The listing builds one solid part. Answer for the finished solid, in the listing's coordinates (mm). Face numbers are marked on the shaded views. A direction names the side the tool comes from. Coordinates: 2 decimals unless noted, no trailing zeros. Order: outer loops, then holes, each group sorted by start corner. A loop starts at its lowest first (then second) coordinate and runs counter-clockwise, first axis right, second up. Notation, with made-up numbers: (42.25, 6.5) -> (76.25, 6.5) arc R19 ccw to (76.25, 10.5) -> close; hole circle Ø9 at (-14, -32). An arc over 180 degrees is marked (long way). Answer in a Markdown table with one row per item.
Autodesk Inventor part; units mm, degrees
ref_plane "YZ Plane" through (0, 0, 0) normal (1, 0, 0) x (0, 1, 0)
ref_plane "XZ Plane" through (0, 0, 0) normal (0, 1, 0) x (-1, 0, 0)
ref_plane "XY Plane" through (0, 0, 0) normal (0, 0, 1) x (1, 0, 0)
sketch "Sketch1" plane through (0, 0, 0) normal (0, 1, 0) x (-1, 0, 0)
  line L0 (-9.6397, 29.7296) -> (10.3603, 29.7296)
  line L1 (12.3603, 29.7296) -> (12.3603, 36.7296)
  line L2 (12.3603, 36.7296) -> (-9.6397, 36.7296)
  line L3 (-9.6397, 36.7296) -> (-9.6397, 29.7296)
  line L4 (12.3603, 36.7296) -> (8.0662, 36.7296)
  line L5 (8.0662, -18.2704) -> (12.3603, -18.2704)
  line L6 (12.3603, -18.2704) -> (-9.6397, -18.2704)
  line L7 (-9.6397, -18.2704) -> (-9.6397, -11.2704)
  line L8 (-9.6397, -11.2704) -> (10.3603, -11.2704)
  line L9 (12.3603, -11.2704) -> (12.3603, -18.2704)
  line L10 (12.3603, -7.7704) -> (22.3603, -7.7704)
  line L11 (22.3603, -7.7704) -> (22.3603, 16.2296)
  line L12 (22.3603, 16.2296) -> (12.3603, 16.2296)
  line L13 (12.3603, -18.2704) -> (12.3603, -7.7704)
  line L14 (12.3603, 16.2296) -> (12.3603, 36.7296)
  line L15 (10.3603, 14.2296) -> (20.3603, 14.2296)
  line L16 (20.3603, 14.2296) -> (20.3603, -5.7704)
  line L17 (20.3603, -5.7704) -> (10.3603, -5.7704)
  line L18 (10.3603, 22.4354) -> (10.3603, 14.2296)
  line L19 (10.3603, -5.7704) -> (10.3603, -4.741)
  line L20 (10.3603, 29.7296) -> (10.3603, 14.2296)
  line L21 (10.3603, -5.7704) -> (10.3603, -11.2704)
  point P0 (0, 0)
  dimension "wall" = 2
  dimension "d1" = 2
  dimension "d2" = 2
  dimension "d3" = 2
  dimension "d4" = 2
  dimension "d5" = 7
  dimension "d6" = 7
  dimension "d7" = 20
  dimension "d8" = 20
  dimension "d9" = 41
  dimension "d10" = 5.5
  dimension "d11" = 20
  dimension "d12" = 10
extrude "Extrusion1" add sketch "Sketch1" along normal blind 10
sketch "Sketch2" plane through (0, 10, 0) normal (0, 1, 0) x (1, 0, 0)
  line L0 (-10.3603, -29.7296) -> (-10.3603, -14.2296) construction
  line L1 (-12.3603, -36.7296) -> (9.6397, -36.7296) construction
  line L2 (9.6397, 18.2704) -> (-12.3603, 18.2704) construction
  line L3 (3.8669, 14.7392) -> (-5.6603, 14.7392) construction
  line L4 (-5.6603, 14.7392) -> (-5.6603, -33.2296) construction
  line L5 (-5.6603, -33.2296) -> (3.8669, -33.2296) construction
  line L6 (3.8669, -33.2296) -> (3.8669, 14.7392) construction
  point P0 (0, 0)
  point P1 (3.8397, -33.2296)
  point P2 (-5.6603, 14.7704)
  dimension "d15" = 4.7
  dimension "d16" = 9.5
  dimension "d17" = 48
  dimension "d18" = 3.5
  dimension "d19" = 3.5
hole "Hole1" at (-5.6603, 10, 33.2296) at (3.8397, 10, 33.2296) at (3.8669, 10, -14.7392) at (-5.6603, 10, -14.7704) direction (0, -1, 0) diameter 1.5 end through all
fillet "Fillet1" radius 2 8 edges at (9.6397, 5, 36.7296) (-12.3603, 5, 36.7296) (9.6397, 5, -18.2704) (-12.3603, 5, -18.2704) (-22.3603, 5, -7.7704) (-12.3603, 5, -7.7704) (-22.3603, 5, 16.2296) (-12.3603, 5, 16.2296)
equation "\"d1\" = wall"
equation "\"d2\" = wall"
equation "\"d3\" = wall"
equation "\"d4\" = wall"
equation "\"d6\" = d5"
equation "\"d8\" = d7"
properties part number "servo_bracket"
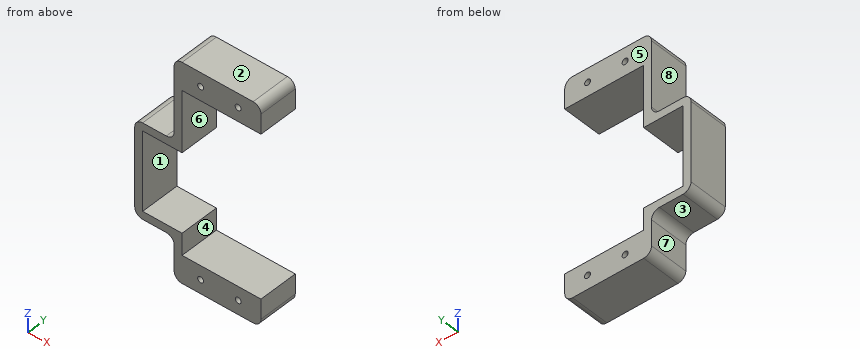
(1) A cutting plane is placed at A-A, the plane x = -19. Determine the outline of the cut face in (y, z).
Check values:
| item | result |
|---|---|
| outline | (0, -7.77) -> (10, -7.77) -> (10, -5.77) -> (0, -5.77) -> close; (0, 14.23) -> (10, 14.23) -> (10, 16.23) -> (0, 16.23) -> close |
(2) Flat-ended cylindrical pins translate along their axes: pin 1 (3 mm diameter, centred on y = 4, z = 7.5, fed in from +X); pin 2 (3 mm diameter, centred on x = -17, y = 5.5, fed in from -Z); pin 3 (1.2 mm diameter, centred on x = -5.66, z = -14.77, fed in from +Y); pin 4 (3 mm diameter, centred on x = -18, y = 3, fed in from +Z). Find the tip coordinate at first contact, or state that the pin passes through.
Check values:
| item | result |
|---|---|
| pin 1 | x = -20.36 |
| pin 2 | z = -7.77 |
| pin 3 | through |
| pin 4 | z = 16.23 |
(3) Find the intervals of material crossed by line 1 along Z through (x, y) = (5, 5.75); line 2 along Z through (x, y) = (-18.5, 2.5); line 3 along X through (y, z) = (3, 33), in increasing order. Write a range as from..to.
Check values:
| item | result |
|---|---|
| line 1 | -18.27..-11.27, 29.73..36.73 |
| line 2 | -7.77..-5.77, 14.23..16.23 |
| line 3 | -12.36..-6.37, -4.95..3.13, 4.55..9.64 |
(4) For a pull along Z with two mould halves and no side action, classify the marked faces 1, 2, 3 and 4 as released by +Z, released by -Z, zero draft, split by the parting line, or undercut.
Check values:
| item | result |
|---|---|
| face 1 | undercut |
| face 2 | released by +Z |
| face 3 | released by -Z |
| face 4 | undercut |
(5) A cutting plane is placed at D-D, the plane z = -12. Determine the outline of the cut face in (x, y), then the cut area to 3 significant figures.
Check values:
| item | result |
|---|---|
| outline | (-12.36, 0) -> (9.64, 0) -> (9.64, 10) -> (-12.36, 10) -> close |
| area | 220 mm² |
(6) A cutting plane is placed at B-B, the plane y = 9. Determine the outline of the cut face in (x, z), then the cut area to 3 significant figures.
Check values:
| item | result |
|---|---|
| outline | (-22.36, -5.77) arc R2 ccw to (-20.36, -7.77) -> (-14.36, -7.77) arc R2 cw to (-12.36, -9.77) -> (-12.36, -16.27) arc R2 ccw to (-10.36, -18.27) -> (7.64, -18.27) arc R2 ccw to (9.64, -16.27) -> (9.64, -11.27) -> (-10.36, -11.27) -> (-10.36, -5.77) -> (-20.36, -5.77) -> (-20.36, 14.23) -> (-10.36, 14.23) -> (-10.36, 29.73) -> (9.64, 29.73) -> (9.64, 34.73) arc R2 ccw to (7.64, 36.73) -> (-10.36, 36.73) arc R2 ccw to (-12.36, 34.73) -> (-12.36, 18.23) arc R2 cw to (-14.36, 16.23) -> (-20.36, 16.23) arc R2 ccw to (-22.36, 14.23) -> close; hole circle Ø1.5 at (-5.66, -14.77); hole circle Ø1.5 at (-5.66, 33.23); hole circle Ø1.5 at (3.84, 33.23); hole circle Ø1.5 at (3.87, -14.74) |
| area | 419 mm² |
(7) Which of the six approach directions +Z, -Z, +X, -X, +Y, -Y give full straight-line access (tool end or side, diameter ignored) to the marked faces 5, 6, 7 and 8?
Check values:
| item | result |
|---|---|
| face 5 | +Z, -Z, +X, -X, +Y |
| face 6 | +X, +Y, -Y |
| face 7 | -Z, -X, +Y, -Y |
| face 8 | +Z, -X, +Y, -Y |
(8) A cutting plane is placed at C-C, the plane x = 1. Determine the outline of the cut face in (y, z), then the cut area to 3 significant figures.
Check values:
| item | result |
|---|---|
| outline | (0, -18.27) -> (10, -18.27) -> (10, -11.27) -> (0, -11.27) -> close; (0, 29.73) -> (10, 29.73) -> (10, 36.73) -> (0, 36.73) -> close |
| area | 140 mm² |
